```python
from build123d import *

# Parameters (mm, degrees)
F0_W      = 3
F0_H      = 8
F1_DEPTH  = 3
F2_DEPTH  = 4.9
F3_DEPTH  = 4.9
F5_DEPTH  = 3
F7_DEPTH  = 3
F8_DEPTH  = 25
F9_DEPTH  = 1
F11_DEPTH = 3
F12_R     = 1.8630386708
F13_DEPTH = 1
F14_R     = 1.9023250727
F15_DEPTH = 1
F16_R     = 1.25
F17_DEPTH = 2
F18_DEPTH = 25


with BuildPart() as f1:
    # F0 (on Top) → F1 (new body)
    with BuildSketch(Plane.XY):
        with BuildLine():
            Line((9.35, -30.6), (9.35, 0))
            ThreePointArc((9.35, 0), (0, -9.35), (-9.35, 0))
            Line((-9.35, 0), (-9.35, -30.6))
            Line((-9.35, -30.6), (9.35, -30.6))
        make_face()
        with Locations((-4.25, -20.6)):
            Rectangle(F0_W, F0_H, mode=Mode.SUBTRACT)
        with Locations((4.25, -20.6)):
            Rectangle(F0_W, F0_H, mode=Mode.SUBTRACT)
        with BuildLine():
            ThreePointArc((-9.35, 0), (0, -9.35), (9.35, 0))
            ThreePointArc((9.35, 0), (0, 9.35), (-9.35, 0))
        make_face()
        with Locations((4.25, -20.6)):
            Rectangle(F0_W, F0_H)
        with Locations((-4.25, -20.6)):
            Rectangle(F0_W, F0_H)
    extrude(amount=-F1_DEPTH)

    # F0 (on Top) → F2 (join)
    with BuildSketch(Plane.XY):
        with Locations((4.25, -20.6)):
            Rectangle(F0_W, F0_H)
    extrude(amount=F2_DEPTH)

    # F0 (on Top) → F3 (join)
    with BuildSketch(Plane.XY):
        with Locations((-4.25, -20.6)):
            Rectangle(F0_W, F0_H)
    extrude(amount=F3_DEPTH)

    # F4 (on face) → F5 (join)
    with BuildSketch(Plane(origin=(-5.75, 0, 0), x_dir=(0, -1, 0), z_dir=(-1, 0, 0))):
        with BuildLine():
            Line((16.6, 4.9), (24.6, 4.9))
            ThreePointArc((24.6, 4.9), (20.6, 8.9), (16.6, 4.9))
        make_face()
    extrude(amount=-F5_DEPTH)

    # F6 (on face) → F7 (join)
    with BuildSketch(Plane.YZ.offset(5.75)):
        with BuildLine():
            Line((-17.944, 4.9), (-16.6, 4.9))
            ThreePointArc((-16.6, 4.9), (-20.6, 8.9), (-24.6, 4.9))
            Line((-24.6, 4.9), (-23.256, 4.9))
            Line((-23.256, 4.9), (-21.928, 7.2001634725))
            Line((-21.928, 7.2001634725), (-19.272, 7.2001634725))
            Line((-19.272, 7.2001634725), (-17.944, 4.9))
        make_face()
        with BuildLine():
            Line((-19.311, 4.9), (-17.944, 4.9))
            Line((-17.944, 4.9), (-19.272, 7.2001634725))
            Line((-19.272, 7.2001634725), (-21.928, 7.2001634725))
            Line((-21.928, 7.2001634725), (-23.256, 4.9))
            Line((-23.256, 4.9), (-21.889, 4.9))
            ThreePointArc((-21.889, 4.9), (-20.6, 6.189), (-19.311, 4.9))
        make_face()
    extrude(amount=-F7_DEPTH)

    # F6 (on face) → F8 (cut)
    with BuildSketch(Plane.YZ.offset(5.75)):
        with BuildLine():
            Line((-21.889, 4.9), (-19.311, 4.9))
            ThreePointArc((-19.311, 4.9), (-20.6, 6.189), (-21.889, 4.9))
        make_face()
        with BuildLine():
            ThreePointArc((-21.889, 4.9), (-20.6, 3.611), (-19.311, 4.9))
            Line((-19.311, 4.9), (-21.889, 4.9))
        make_face()
    extrude(amount=-F8_DEPTH, mode=Mode.SUBTRACT)

    # F6 (on face) → F9 (cut)
    with BuildSketch(Plane.YZ.offset(5.75)):
        with BuildLine():
            Line((-19.311, 4.9), (-17.944, 4.9))
            Line((-17.944, 4.9), (-19.272, 7.2001634725))
            Line((-19.272, 7.2001634725), (-21.928, 7.2001634725))
            Line((-21.928, 7.2001634725), (-23.256, 4.9))
            Line((-23.256, 4.9), (-21.889, 4.9))
            ThreePointArc((-21.889, 4.9), (-20.6, 6.189), (-19.311, 4.9))
        make_face()
        with BuildLine():
            Line((-19.272, 2.5998365275), (-17.944, 4.9))
            Line((-17.944, 4.9), (-19.311, 4.9))
            ThreePointArc((-19.311, 4.9), (-20.6, 3.611), (-21.889, 4.9))
            Line((-21.889, 4.9), (-23.256, 4.9))
            Line((-23.256, 4.9), (-21.928, 2.5998365275))
            Line((-21.928, 2.5998365275), (-19.272, 2.5998365275))
        make_face()
    extrude(amount=-F9_DEPTH, mode=Mode.SUBTRACT)

    # F10 (on face) → F11 (join)
    with BuildSketch(Plane.XY):
        with BuildLine():
            Line((9.85, -31.1), (9.85, 0))
            ThreePointArc((9.85, 0), (0, 9.85), (-9.85, 0))
            Line((-9.85, 0), (-9.85, -31.1))
            Line((-9.85, -31.1), (9.85, -31.1))
        make_face()
        with BuildLine():
            Line((-9.35, -30.6), (-9.35, 0))
            ThreePointArc((-9.35, 0), (0, 9.35), (9.35, 0))
            Line((9.35, 0), (9.35, -30.6))
            Line((9.35, -30.6), (-9.35, -30.6))
        make_face(mode=Mode.SUBTRACT)
    extrude(amount=-F11_DEPTH)

    # F12 (on face) → F13 (join)
    with BuildSketch(Plane.YZ.offset(-2.75)):
        with Locations((-20.6, 4.9)):
            Circle(F12_R)
    extrude(amount=-F13_DEPTH)

    # F14 (on face) → F15 (join)
    with BuildSketch(Plane(origin=(2.75, 0, 0), x_dir=(0, -1, 0), z_dir=(-1, 0, 0))):
        with Locations((20.6, 4.9)):
            Circle(F14_R)
    extrude(amount=-F15_DEPTH)

    # F16 (on face) → F17 (join)
    with BuildSketch(Plane.XY):
        with Locations((6.65, -3.1)):
            Circle(F16_R)
    extrude(amount=F17_DEPTH)

    # F18 (cut): a face of the model
    f18_faces = [f1.faces().sort_by_distance(p)[0] for p in [
        (-3.75, -20.6, 4.9),
    ]]
    extrude(f18_faces, amount=-F18_DEPTH, mode=Mode.SUBTRACT)


solid = f1.part
```
Design review of the part built by this model. Coordinates are the model's own, in mm. A direction names the side the tool comes from. Round coordinates to 2 decimals unless told otherwise and drop trailing zeros. Order: outer loops, then holes, each group sorted by start corner. A loop starts at its lowest first (then second) coordinate and runs counter-clockwise, first axis right, second up. Notation, with made-up numbers: (7.25, 2.5) - (18.25, 2.5) arc R17 ccw to (18.25, 29.5) - close; hole circle Ø9 at (68.5, 35.25). An arc over 180 degrees is marked (long way). Return JSON: item names as keys, results as strings.
Q1. For pin 1 Ø2 at (y, z) = (-3.5, 3.5) entering from -X; pin 2 Ø0.9 at (x, z) = (-3.5, 2) entering from -Y; pin 3 Ø2 at (x, z) = (6.5, 2) entering from +Y; pin 4 Ø4 at (y, z) = (-20.6, 4.9) entering from -X, all flat-tipped, find the tip position at first contact; note any pin that passes through.
Computed values:
{"pin 1": "passes through", "pin 2": "stops at y = -24.6", "pin 3": "stops at y = -1.85", "pin 4": "stops at x = -5.75"}
Q2. Consider section A-A on y = -20.6. Write out the cut boundary in (x, z).
Computed values:
{"outline": "(-9.85, -3) - (9.85, -3) - (9.85, 0) - (5.75, 0) - (5.75, 2.6) - (4.75, 2.6) - (4.75, 3.61) - (2.75, 3.61) - (2.75, 0) - (-2.75, 0) - (-2.75, 3.61) - (-5.75, 3.61) - (-5.75, 0) - (-9.85, 0) - close; (-5.75, 6.19) - (-2.75, 6.19) - (-2.75, 8.9) - (-5.75, 8.9) - close; (2.75, 6.19) - (4.75, 6.19) - (4.75, 7.2) - (5.75, 7.2) - (5.75, 8.9) - (2.75, 8.9) - close"}
Q3. Wall thickness on L1, parallel to X at y = -19, z = 6.25; L2, parallel to Z at x = -4.85, y = -20.6; L3, parallel to Z at x = 1.5, y = -16: over which ranges is each line inside the solid? List them lowest first. Write a range as [from, to].
Computed values:
{"L1": "x = [-5.75, -2.75], [2.75, 4.75]", "L2": "z = [-3, 3.61], [6.19, 8.9]", "L3": "z = [-3, 0]"}
Q4. Consider section C-C on x = -5. Write out the cut boundary in (y, z).
Computed values:
{"outline": "(-31.1, -3) - (8.49, -3) - (8.49, 0) - (-16.6, 0) - (-16.6, 4.9) arc R4 ccw to (-24.6, 4.9) - (-24.6, 0) - (-31.1, 0) - close; hole circle Ø2.58 at (-20.6, 4.9)"}
Q5. Consider section D-D on y = -3.1. Write out the cut boundary in (x, z), plus the area to 3 significant figures.
Computed values:
{"outline": "(-9.85, -3) - (9.85, -3) - (9.85, 0) - (7.9, 0) - (7.9, 2) - (5.4, 2) - (5.4, 0) - (-9.85, 0) - close", "area": "64.1 mm2"}
Q6. Consider section B-B on z = 0.75. Write out the cut boundary in (x, y).
Computed values:
{"outline": "(-5.75, -24.6) - (-2.75, -24.6) - (-2.75, -16.6) - (-5.75, -16.6) - close; (2.75, -24.6) - (5.75, -24.6) - (5.75, -16.6) - (2.75, -16.6) - close; circle Ø2.5 at (6.65, -3.1)"}
Q7. The part is to be moulded in two halves that separate along Y. For faces 1 (the flat face through (-9.85, -15, -1)), 2 (the flat face through (4, -24.6, 2)), 3 (the flat face through (5.26, -18.62, 3.73)), say which applies: pulls with the +Y half, pulls with the -Y half, needs draft (parallel to the pull), parting line crosses it, or undercut.
Computed values:
{"face 1": "needs draft", "face 2": "pulls with the -Y half", "face 3": "undercut"}
Q8. Machinability: for faces 4 (the flat face through (5.75, -22.4, 2.5)), 5 (the flat face through (5.257, -22.601, 3.766)), 6 (the flat face through (-4, -16.6, 2)), which of the approach directions +Z, -Z, +X, -X, +Y, -Y give a long, thin tool a straight path to every point of the face, cutting with its end or side? Answer none if there is none.
Computed values:
{"face 4": "+Z, +X, -Y", "face 5": "+X", "face 6": "+Z, +X, -X, +Y"}
